Part model, mm, in its own coordinate system. Round coordinates to 2 decimals unless told otherwise and drop trailing zeros. Order: outer loops, then holes, each group sorted by start corner. A loop starts at its lowest first (then second) coordinate and runs counter-clockwise, first axis right, second up. Notation, with made-up numbers: M 16.5,30 L 27.5,30 A15 cw 27.5,34 Z; hole C 22.5,47.25 d6. An arc over 180 degrees is marked long. Write each question's results on one line, items separated by ' | '. Start each with the question number.
1. Band-saw the part on C-C, the plane x = -112.5. List the corners of the cut face in (y, z).
2. Band-saw the part on B-B, the plane z = 5.25. Give the number of separate pieces and of enclosed holes in the cut face, then the cut area to 3 significant figures.
3. Probe L1, parallel to Y at x = -42.5, z = 6; L2, parallel to Y at x = -144, z = 2; L3, parallel to X at y = 27.5, z = 6.25 (3 decimals). List the from-to ranges inside material, lowest first. Write a range as [from, to].
4. Band-saw the part on A-A, the plane y = -17.5. List the corners of the cut face in (x, z).
5. Drop a flat-ended pin along its axis: pin 1 Ø1 at (y, z) = (37.5, 2) entering from -X. Give the stop position or say it passes through.
6. Band-saw the part on D-D, the plane y = 48. List the corners of the cut face in (x, z), then the cut area to 3 significant figures.
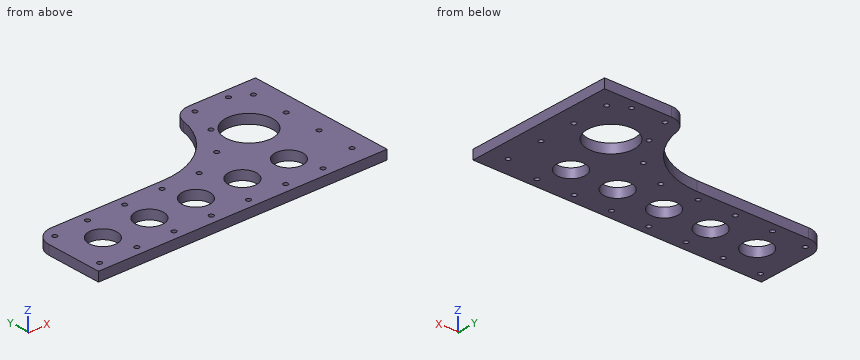
Autodesk Inventor part; units mm, degrees
ref_plane "YZ Plane" through (0, 0, 0) normal (1, 0, 0) x (0, 1, 0)
ref_plane "XZ Plane" through (0, 0, 0) normal (0, 1, 0) x (-1, 0, 0)
ref_plane "XY Plane" through (0, 0, 0) normal (0, 0, 1) x (1, 0, 0)
sketch "Sketch1" plane through (0, 0, 0) normal (0, 0, 1) x (1, 0, 0)
  line L0 (-175.7553, 1.949) -> (-175.7553, -36.151)
  line L1 (-175.7553, -36.151) -> (21.0947, -36.151)
  line L2 (21.0947, -36.151) -> (21.0947, 65.449)
  line L3 (21.0947, 65.449) -> (-36.0553, 65.449)
  line L4 (-163.0553, 14.649) -> (-86.8553, 14.649)
  line L5 (-36.0553, 65.449) -> (-36.0553, 65.449)
  arc A0 (-86.8553, 14.649) -> (-36.0553, 65.449) centre (-86.8553, 65.449) ccw
  arc A1 (-163.0553, 14.649) -> (-175.7553, 1.949) centre (-163.0553, 1.949) ccw
  point P0 (0, 0)
  point P1 (-175.7553, 14.649)
  dimension "d0" = 196.85
  dimension "d1" = 101.6
  dimension "d2" = 57.15
  dimension "d3" = 50.8
  dimension "d7" = 50.8
  dimension "d8" = 12.7
extrude "Extrusion1" add sketch "Sketch1" along normal blind 6.35
hole "Hole1" at (-169.4053, -29.801, 6.35) direction (0, 0, -1) diameter 3.175 end through all
pattern_linear "Rectangular Pattern1" count 7 spacing 25.4 along (1, 0, 0) of "Hole1"
hole "Hole2" at (-144.0053, 8.299, 6.35) direction (0, 0, -1) diameter 3.175 end through all
pattern_linear "Rectangular Pattern2" count 4 spacing 25.4 along (1, 0, 0) of "Hole2"
hole "Hole3" at (-46.2174, 19.2208, 6.35) direction (0, 0, -1) diameter 3.175 end through all
hole "Hole4" at (-32.5291, 39.1356, 6.35) direction (0, 0, -1) diameter 3.175 end through all
hole "Hole5" at (-25.8953, 59.099, 6.35) direction (0, 0, -1) diameter 3.175 end through all
pattern_linear "Rectangular Pattern3" count 2 spacing 22.86 along (1, 0, 0) of "Hole5"
hole "Hole6" at (-167.6661, 6.7836, 6.35) direction (0, 0, -1) diameter 3.175 end through all
fillet "Fillet1" radius 12.7 1 edges at (-36.0553, 65.449, 3.175)
hole "Hole7" at (-150.3553, -10.751, 6.35) direction (0, 0, -1) diameter 19.05 end through all
pattern_linear "Rectangular Pattern4" count 5 spacing 31.75 along (1, 0, 0) of "Hole7"
hole "Hole8" at (-17.0053, 27.349, 6.35) direction (0, 0, -1) diameter 31.75 end through all
hole "Hole9" at (8.3947, -23.451, 6.35) direction (0, 0, -1) diameter 3.175 end through all
pattern_linear "Rectangular Pattern5" count 4 spacing 25.4 along (0, 1, 0) of "Hole9"
properties part number "arm droit"
Solution:
1) outline: M -36.15,0 L -18.06,0 L -18.06,6.35 L -36.15,6.35 Z; M -3.44,0 L 14.65,0 L 14.65,6.35 L -3.44,6.35 Z
2) separate pieces: 1 | enclosed holes: 26 | area: 11,000 mm^2
3) L1: [-36.15, -31.39], [-28.22, 40.69] | L2: [-36.15, -31.39], [-28.21, -17.85], [-3.66, 6.71], [9.89, 14.65] | L3: [-53.084, -32.88], [-1.131, 6.814], [9.975, 21.095]
4) outline: M -175.76,0 L -157.08,0 L -157.08,6.35 L -175.76,6.35 Z; M -143.63,0 L -125.33,0 L -125.33,6.35 L -143.63,6.35 Z; M -111.88,0 L -93.58,0 L -93.58,6.35 L -111.88,6.35 Z; M -80.13,0 L -61.83,0 L -61.83,6.35 L -80.13,6.35 Z; M -48.38,0 L -30.08,0 L -30.08,6.35 L -48.38,6.35 Z; M -16.63,0 L 21.09,0 L 21.09,6.35 L -16.63,6.35 Z
5) pin 1: x = -44.77
6) outline: M -39.15,0 L 21.09,0 L 21.09,6.35 L -39.15,6.35 Z | area: 383 mm^2
